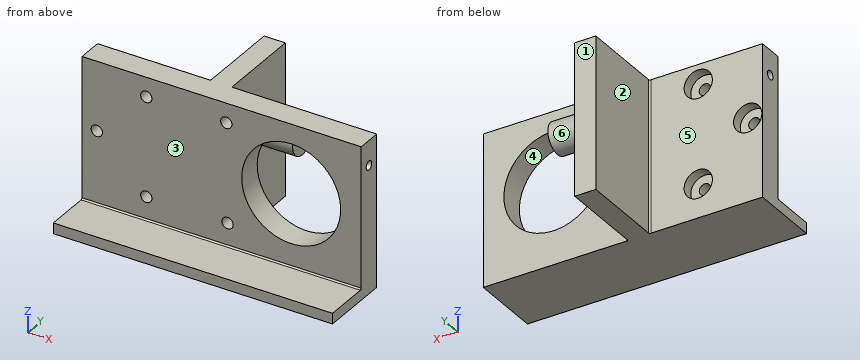
```python
from build123d import *

# Parameters (mm, degrees)
SKETCH_1_W               = 39.5
SKETCH_1_H               = 3.5
EXTRUDE_1_DEPTH          = 19.5
CUT_EXTRUDE_1_REACH      = 44.062
SKETCH_3_R               = 7
EXTRUDE_START            = -3.5
SKETCH_4_W               = 39.5
SKETCH_4_H               = 2
EXTRUDE_2_DEPTH          = 10
CUT_EXTRUDE_2_REACH      = 45.092
SKETCH_5_R               = 0.8
HOLE_WIZARD_M1_6_1_D     = 1.25
HOLE_WIZARD_M1_6_1_DEPTH = 4.15
HOLE_WIZARD_M1_6_1_TIP   = 0.375537887
HOLE_WIZARD_M1_6_2_D     = 1.25
HOLE_WIZARD_M1_6_2_DEPTH = 4.15
HOLE_WIZARD_M1_6_2_TIP   = 0.375537887
SKETCH_10_W              = 21.5
SKETCH_10_H              = 12.103276992
EXTRUDE_3_DEPTH          = 3
SKETCH_11_R              = 2.2
EXTRUDE_4_DEPTH          = 5
SKETCH_12_W              = 39.5
SKETCH_12_H              = 0.5
CUT_EXTRUDE_3_DEPTH      = 6.5
FILLET_1_R               = 0.2
FILLET_2_R               = 0.2
SKETCH_13_R              = 2
CUT_EXTRUDE_4_DEPTH      = 1.5


with BuildPart() as part:
    # 草图1 → 凸台-拉伸1 (new body)
    with BuildSketch(Plane.XY):
        with Locations((-17.354026846, 0.57630481)):
            Rectangle(SKETCH_1_W, SKETCH_1_H)
    extrude(amount=EXTRUDE_1_DEPTH)

    # 草图3 → 切除-拉伸1 (cut, up to next)
    with BuildSketch(Plane(origin=(0, 2.32630481, 0), x_dir=(1, 0, 0), z_dir=(0, 1, 0)), mode=Mode.PRIVATE) as cut_extrude_1_sk1:
        with Locations(Location((-7.514026846, -9.75, 0), (0, 0, 270))):
            Circle(SKETCH_3_R)
    cut_extrude_1_tool1 = extrude(cut_extrude_1_sk1.sketch, amount=-CUT_EXTRUDE_1_REACH, mode=Mode.PRIVATE) & part.part
    add(cut_extrude_1_tool1.solids().sort_by_distance((-7.514027, 2.326305, 9.75))[0], mode=Mode.SUBTRACT)

    # 草图4 → 凸台-拉伸2 (add)
    with BuildSketch(Plane.XZ.offset(1.17369519).offset(EXTRUDE_START)):
        with Locations((-17.354026846, -1)):
            Rectangle(SKETCH_4_W, SKETCH_4_H)
    extrude(amount=EXTRUDE_2_DEPTH)

    # 草图5 → 切除-拉伸2 (cut, up to next)
    with BuildSketch(Plane(origin=(0, 2.32630481, 0), x_dir=(1, 0, 0), z_dir=(0, 1, 0)), mode=Mode.PRIVATE) as cut_extrude_2_sk1:
        with Locations(Location((-35.014026846, -9.75, 0), (0, 0, 270))):
            Circle(SKETCH_5_R)
    cut_extrude_2_tool1 = extrude(cut_extrude_2_sk1.sketch, amount=-CUT_EXTRUDE_2_REACH, mode=Mode.PRIVATE) & part.part
    # 草图5 → 切除-拉伸2 (cut, up to next)
    with BuildSketch(Plane(origin=(0, 2.32630481, 0), x_dir=(1, 0, 0), z_dir=(0, 1, 0)), mode=Mode.PRIVATE) as cut_extrude_2_sk2:
        with Locations(Location((-28.014026846, -2.75, 0), (0, 0, 270))):
            Circle(SKETCH_5_R)
    cut_extrude_2_tool2 = extrude(cut_extrude_2_sk2.sketch, amount=-CUT_EXTRUDE_2_REACH, mode=Mode.PRIVATE) & part.part
    # 草图5 → 切除-拉伸2 (cut, up to next)
    with BuildSketch(Plane(origin=(0, 2.32630481, 0), x_dir=(1, 0, 0), z_dir=(0, 1, 0)), mode=Mode.PRIVATE) as cut_extrude_2_sk3:
        with Locations(Location((-28.014026846, -16.75, 0), (0, 0, 270))):
            Circle(SKETCH_5_R)
    cut_extrude_2_tool3 = extrude(cut_extrude_2_sk3.sketch, amount=-CUT_EXTRUDE_2_REACH, mode=Mode.PRIVATE) & part.part
    # 草图5 → 切除-拉伸2 (cut, up to next)
    with BuildSketch(Plane(origin=(0, 2.32630481, 0), x_dir=(1, 0, 0), z_dir=(0, 1, 0)), mode=Mode.PRIVATE) as cut_extrude_2_sk4:
        with Locations(Location((-16.514026846, -2.75, 0), (0, 0, 270))):
            Circle(SKETCH_5_R)
    cut_extrude_2_tool4 = extrude(cut_extrude_2_sk4.sketch, amount=-CUT_EXTRUDE_2_REACH, mode=Mode.PRIVATE) & part.part
    # 草图5 → 切除-拉伸2 (cut, up to next)
    with BuildSketch(Plane(origin=(0, 2.32630481, 0), x_dir=(1, 0, 0), z_dir=(0, 1, 0)), mode=Mode.PRIVATE) as cut_extrude_2_sk5:
        with Locations(Location((-16.694026846, -16.75, 0), (0, 0, 270))):
            Circle(SKETCH_5_R)
    cut_extrude_2_tool5 = extrude(cut_extrude_2_sk5.sketch, amount=-CUT_EXTRUDE_2_REACH, mode=Mode.PRIVATE) & part.part
    add(cut_extrude_2_tool1.solids().sort_by_distance((-35.014027, 2.326305, 9.75))[0], mode=Mode.SUBTRACT)
    add(cut_extrude_2_tool2.solids().sort_by_distance((-28.014027, 2.326305, 2.75))[0], mode=Mode.SUBTRACT)
    add(cut_extrude_2_tool3.solids().sort_by_distance((-28.014027, 2.326305, 16.75))[0], mode=Mode.SUBTRACT)
    add(cut_extrude_2_tool4.solids().sort_by_distance((-16.514027, 2.326305, 2.75))[0], mode=Mode.SUBTRACT)
    add(cut_extrude_2_tool5.solids().sort_by_distance((-16.694027, 2.326305, 16.75))[0], mode=Mode.SUBTRACT)

    # M1.6 螺纹孔1
    with Locations(Plane.ZY.offset(37.104026846)):
        with Locations((16, 0.57630481)):
            Hole(HOLE_WIZARD_M1_6_1_D / 2, depth=HOLE_WIZARD_M1_6_1_DEPTH)
            with Locations((0, 0, -(HOLE_WIZARD_M1_6_1_DEPTH + HOLE_WIZARD_M1_6_1_TIP / 2))):  # 118° drill point
                Cone(0, HOLE_WIZARD_M1_6_1_D / 2, HOLE_WIZARD_M1_6_1_TIP, mode=Mode.SUBTRACT)

    # M1.6 螺纹孔2
    with Locations(Plane(origin=(2.395973154, 0, 0), x_dir=(0, 0, -1), z_dir=(1, 0, 0))):
        with Locations((-16, 0.57630481)):
            Hole(HOLE_WIZARD_M1_6_2_D / 2, depth=HOLE_WIZARD_M1_6_2_DEPTH)
            with Locations((0, 0, -(HOLE_WIZARD_M1_6_2_DEPTH + HOLE_WIZARD_M1_6_2_TIP / 2))):  # 118° drill point
                Cone(0, HOLE_WIZARD_M1_6_2_D / 2, HOLE_WIZARD_M1_6_2_TIP, mode=Mode.SUBTRACT)

    # 草图10 → 凸台-拉伸3 (add)
    with BuildSketch(Plane.ZY.offset(18.104026846)):
        with Locations((8.75, 8.377943306)):
            Rectangle(SKETCH_10_W, SKETCH_10_H)
    extrude(amount=EXTRUDE_3_DEPTH)

    # 草图11 → 凸台-拉伸4 (add)
    with BuildSketch(Plane.ZY.offset(18.104026846)):
        with Locations((9.75, 10.299581802)):
            Circle(SKETCH_11_R)
    extrude(amount=-EXTRUDE_4_DEPTH)

    # 草图12 → 切除-拉伸3 (cut)
    with BuildSketch(Plane.XZ.offset(7.67369519)):
        with Locations((-17.354026846, -0.25)):
            Rectangle(SKETCH_12_W, SKETCH_12_H)
    extrude(amount=-CUT_EXTRUDE_3_DEPTH, mode=Mode.SUBTRACT)

    # 圆角1
    fillet_1_edges = [part.edges().sort_by_distance(p)[0] for p in [
        (-17.354026846, -1.17369519, -0.5),
    ]]
    fillet(fillet_1_edges, radius=FILLET_1_R)

    # 圆角2
    fillet_2_edges = [part.edges().sort_by_distance(p)[0] for p in [
        (-18.104026846, 2.32630481, 8.75),
        (-21.104026846, 2.32630481, 8.75),
    ]]
    fillet(fillet_2_edges, radius=FILLET_2_R)

    # 草图13 → 切除-拉伸4 (cut)
    with BuildSketch(Plane(origin=(0, 2.32630481, 0), x_dir=(1, 0, 0), z_dir=(0, 1, 0))):
        with Locations(Location((-28.014026846, -2.75, 0), (0, 0, 270))):
            Circle(SKETCH_13_R)
        with Locations(Location((-28.014026846, -16.75, 0), (0, 0, 270))):
            Circle(SKETCH_13_R)
        with Locations(Location((-35.014026846, -9.75, 0), (0, 0, 270))):
            Circle(SKETCH_13_R)
    extrude(amount=-CUT_EXTRUDE_4_DEPTH, mode=Mode.SUBTRACT)


solid = part.part
```
Part model, mm, in its own coordinate system. Face numbers are marked on the shaded views. A direction names the side the tool comes from. Round coordinates to 2 decimals unless told otherwise and drop trailing zeros. Loops run counter-clockwise (first coordinate to the right, second up) from the corner with the lowest first, then second, coordinate; pieces in that order, holes last.
Item 1: Drill centre lines: line 1 (X direction, y = 0.1, z = 9.75); line 2 (Y direction, x = -35.2, z = 16); line 3 (X direction, y = 8.25, z = 7). Where is each one in solid material? Low to high.
Item 2: Cut at A-A, the plane z = 9.75. Give the cut face in (x, y).
Item 3: Cut at B-B, the plane z = 6. Give the cut face in (x, y), then the cut area to 3 significant figures.
Item 4: Cut at D-D, the plane y = 9.5. Give the cut face in (x, z).
Item 5: 3-axis set-ups, long thin cutter, end or side, ignore diameter. For the marked faces 1, 2 and 3: which of +Z, -Z, +X, -X, +Y, -Y reach the whole face in a straight line?
Item 6: Mould opens along Y. For the marked faces 4, 5 and 6 say: +Y half, -Y half, draft (parallel to the pull), parting line (faces both ways), or undercut.
Item 7: Cut at C-C, the plane y = 3. Give the cut face in (x, z).
Item 8: Drop flat-ended pins along their axis: P1, Ø0.8, axis at y = 0.58, z = 16, coming from the +X side; P2, Ø2, axis at x = -28.01, z = 16.75, coming from the +Y side; P3, Ø8, axis at x = -13.5, z = 12.5, coming from the +Y side; P4, Ø4, axis at y = -4, z = 2.5, coming from the -X side. Give the stop position or say it passes through.
A:
1. line 1: x = -37.1 to -35.81, -34.21 to -14.51, -0.51 to 2.4
1. line 2: y = -1.17 to -0.05, 1.2 to 2.33
1. line 3: x = -21.1 to -18.1
2. outline: (-37.1, -1.17) - (-35.81, -1.17) - (-35.81, 0.83) - (-37.01, 0.83) - (-37.01, 2.33) - (-37.1, 2.33) - close; (-34.21, -1.17) - (-14.51, -1.17) - (-14.51, 2.33) - (-17.9, 2.33) arc R0.2 cw to (-18.1, 2.53) - (-18.1, 8.1) - (-13.1, 8.1) - (-13.1, 12.5) - (-18.1, 12.5) - (-18.1, 14.43) - (-21.1, 14.43) - (-21.1, 2.53) arc R0.2 cw to (-21.3, 2.33) - (-33.01, 2.33) - (-33.01, 0.83) - (-34.21, 0.83) - close; (-0.51, -1.17) - (2.4, -1.17) - (2.4, 2.33) - (-0.51, 2.33) - close
3. outline: (-37.1, -1.17) - (-13.42, -1.17) - (-13.42, 2.33) - (-17.9, 2.33) arc R0.2 cw to (-18.1, 2.53) - (-18.1, 14.43) - (-21.1, 14.43) - (-21.1, 2.53) arc R0.2 cw to (-21.3, 2.33) - (-37.1, 2.33) - close; (-1.6, -1.17) - (2.4, -1.17) - (2.4, 2.33) - (-1.6, 2.33) - close
3. area: 133 mm2
4. outline: (-21.1, -2) - (-18.1, -2) - (-18.1, 7.7) - (-13.1, 7.7) - (-13.1, 11.8) - (-18.1, 11.8) - (-18.1, 19.5) - (-21.1, 19.5) - close
5. face 1: +Z, -Z, +X, -X, +Y
5. face 2: +Z, -Z, -X, +Y
5. face 3: +Z, +X, -X, -Y
6. face 4: draft
6. face 5: +Y half
6. face 6: undercut
7. outline: (-21.1, -2) - (-18.1, -2) - (-18.1, 19.5) - (-21.1, 19.5) - close
8. P1: stops at x = -1.89
8. P2: stops at y = 0.83
8. P3: stops at y = 12.5
8. P4: passes through
